from build123d import *

# Parameters (mm, degrees)
F1_DEPTH    = 5
F2_T1_DEPTH = 5
F2_T3_DEPTH = 27.4743818089
F3_R        = 28.9973991458
F4_R        = 14.3918110757


# Not quite as in the source:
# - a fillet or chamfer that OpenCascade refuses, or shapes differently, is made with other operations: its cross-section is extruded or revolved along the edge and cut away or added


with BuildPart() as f1:
    # F0 (on Top) → F1 (new body)
    with BuildSketch(Plane.XY):
        Polygon((-25, 0), (0, 0), (0, -62.5), (1.0401320628, -59.1675673885), (11, 0), (11, 17), (7, 17), (0, 5), (-25, 5), (-37, -3), (-25, -3), align=None)
    extrude(amount=F1_DEPTH)

    # F2: fillet of radius 7.861186634 on 2 edges, made by hand

    # F2_s2 → F2_t1 (join)
    with BuildSketch(Plane.XY):
        with BuildLine():
            ThreePointArc((2.27509477, 8.9001624629), (-0.5998840547, 6.0444203344), (-4.5152323805, 5))
            Line((-4.5152323805, 5), (0, 5))
            Line((0, 5), (2.27509477, 8.9001624629))
        make_face()
    extrude(amount=F2_T1_DEPTH)

    # F2_s4 → F2_t3 (cut)
    with BuildSketch(Plane.XY.offset(-11.2371909045)):
        with BuildLine():
            ThreePointArc((11, 17), (7.3843664174, 15.838413937), (4.735162038, 13.1174206365))
            Line((4.735162038, 13.1174206365), (7, 17))
            Line((7, 17), (11, 17))
        make_face()
    extrude(amount=F2_T3_DEPTH, mode=Mode.SUBTRACT)

    # F3
    f3_edges = [f1.edges().sort_by_distance(p)[0] for p in [
        (-25, 5, 2.5),
    ]]
    fillet(f3_edges, radius=F3_R)

    # F4
    f4_edges = [f1.edges().sort_by_distance(p)[0] for p in [
        (1.040132, -59.167567, 2.5),
    ]]
    fillet(f4_edges, radius=F4_R)


solid = f1.part
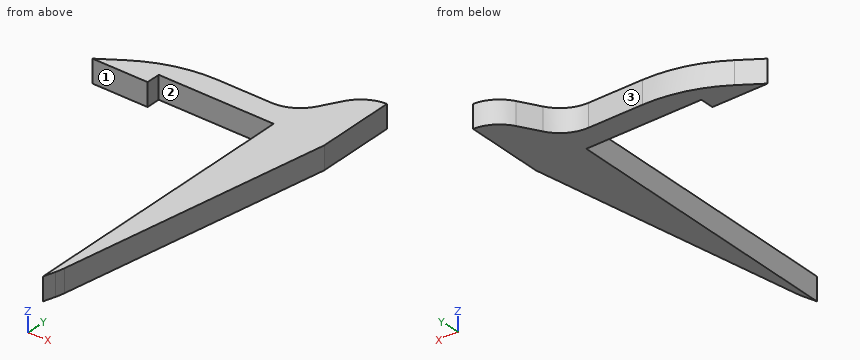
Model file for the job. Use its own axes, mm. Face numbers are marked on the shaded views. A direction names the side the tool comes from. Give positions to 0.01 mm unless a question says otherwise; leave off trailing zeros. Loops run counter-clockwise (first coordinate to the right, second up) from the corner with the lowest first, then second, coordinate; pieces in that order, holes last.
1) Wall check: line 1 (Y direction, x = -4, z = 2.1); line 2 (Y direction, x = -28.5, z = 2.5); line 3 (X direction, y = -30.5, z = 1.4). Give the ranges that are in metal, low to high.
2) Flat gauge pins, fed straight in: pin 1 Ø3 at (y, z) = (-48.5, 1.5) entering from -X; pin 2 Ø2.5 at (x, z) = (-9, 1.5) entering from -Y; pin 3 Ø3 at (y, z) = (-2, 1.5) entering from +X. Where does each tip first touch, or does it go through?
3) Saw through at A-A (z = 1.1). Write the cut outline in (x, y).
4) Saw through at B-B (y = -30). Write the cut outline in (x, z), plus the area to 4 significant figures.
5) Saw through at C-C (x = -7.5). Write the cut outline in (y, z), plus the area to 3 significant figures.
6) Tool access for the marked faces 1, 2 and 3: list every direction of +Z, -Z, +X, -X, +Y, -Y with a clear straight run to the whole face (end or side of a thin tool).
Answer block:
1. line 1: y = 0 to 5.02
1. line 2: y = -3 to 2.27
1. line 3: x = 0 to 5.87
2. pin 1: stops at x = 0
2. pin 2: stops at y = 0
2. pin 3: stops at x = 10.92
3. outline: (-37, -3) - (-25, -3) - (-25, 0) - (0, 0) - (0, -62.5) - (0.75, -60.1) arc R14.39 ccw to (1.2, -58.2) - (11, 0) - (11, 17) arc R7.86 ccw to (4.74, 13.12) - (2.28, 8.9) arc R7.86 cw to (-4.52, 5) - (-16.22, 5) arc R29 ccw to (-32.31, 0.13) - close
4. outline: (0, 0) - (5.95, 0) - (5.95, 5) - (0, 5) - close
4. area: 29.75 mm2
5. outline: (0, 0) - (5, 0) - (5, 5) - (0, 5) - close
5. area: 25.0 mm2
6. face 1: +Z, -Z, -X, -Y
6. face 2: +Z, -Z, -Y
6. face 3: +Z, -Z, -X, +Y
